Autodesk Inventor part; units mm, degrees
ref_plane "YZ Plane" through (0, 0, 0) normal (1, 0, 0) x (0, 1, 0)
ref_plane "XZ Plane" through (0, 0, 0) normal (0, 1, 0) x (-1, 0, 0)
ref_plane "XY Plane" through (0, 0, 0) normal (0, 0, 1) x (1, 0, 0)
sketch "Sketch1" plane through (0, 0, 0) normal (0, 1, 0) x (-1, 0, 0)
  circle A0 centre (0, 0) radius 53.71
  circle A1 centre (0, 0) radius 50.71
  dimension "d0" = 107.42
  dimension "d1" = 3
extrude "Extrusion1" add sketch "Sketch1" along normal blind 30
sketch "Sketch2" plane through (0, 0, 0) normal (0, -1, 0) x (1, 0, 0)
  circle A0 centre (0, 0) radius 53.71
  circle A1 centre (0, 0) radius 50.71
  circle A2 centre (0, 0) radius 40.71
  dimension "d5" = 10
extrude "Extrusion2" add sketch "Sketch2" along normal blind 3 contours A0 | A1
properties part number "12mm-CoilForm-Stiffner"
The listing builds one solid part. Answer for the finished solid, in the listing's coordinates (mm). A direction names the side the tool comes from. Round coordinates to 2 decimals unless told otherwise and drop trailing zeros. Write each loop counter-clockwise with the first axis right and the second up, starting at its lowest first coordinate (ties: lowest second). Pieces come first, ordered by that corner, then holes. Notation, with made-up numbers: (-36.5, 43.25) - (-8.5, 43.25) arc R18 ccw to (-8.5, 77.25) - close; hole circle Ø1 at (69, 0.25). An arc over 180 degrees is marked (long way). Use one line per item in the form item = value. Start each with the question number.
Item 1: A tool of negligible diameter and unlimited length cuts with its end or side. For faces 1 (the flat face through (-40, 30, 32)), 2 (the flat face through (0, 0, 42)), from which of +Z, -Z, +X, -X, +Y, -Y can it reach the whole face along a straight path? Write none if from no direction.
Item 2: Flat-ended cylindrical pins translate along their axes: pin 1 Ø10 at (y, z) = (19, 27.5) entering from +X; pin 2 Ø4 at (x, y) = (42, 11.5) entering from +Z; pin 3 Ø10 at (x, y) = (-42.5, 23) entering from -Z. Find the tip coordinate at first contact, or state that the pin passes through.
Item 3: A cutting plane is placed at D-D (x = -47). Write down the section's boundary in (y, z), plus the area to 3 significant figures.
Item 4: A cutting plane is placed at B-B (x = 0). Write down the section's boundary in (y, z).
Item 5: Determine the mould class of faces 3 (the flat face through (-8.21, -3, 40.04)), 4 (the cylindrical face through (38.83, -1.48, -12.23)) for opening direction Z: +Z half, -Z half, draft (parallel to the pull), parting line (faces both ways), or undercut.
Item 6: Find the intervals of material crossed by line 1 (Z direction, x = 0, y = -1.15); line 2 (Z direction, x = 0, y = 10); line 3 (Y direction, x = -4.5, z = -40.5), in increasing order. Write a range as [from, to].
Item 7: A cutting plane is placed at C-C (y = 25.5). Write down the section's boundary in (x, z), plus the area to 3 significant figures.
Item 8: A cutting plane is placed at A-A (z = 0). Write down the section's boundary in (x, y), plus the area to 3 significant figures.
The answers:
q1.face_1 = +Z, -Z, +X, -X, +Y
q1.face_2 = +Y
q2.pin_1 = 48.77
q2.pin_2 = 35.84
q2.pin_3 = -38.45
q3.outline = (-3, -26) - (30, -26) - (30, -19.04) - (0, -19.04) - (0, 19.04) - (30, 19.04) - (30, 26) - (-3, 26) - close
q3.area = 573 mm^2
q4.outline = (-3, -53.71) - (30, -53.71) - (30, -50.71) - (0, -50.71) - (0, -40.71) - (-3, -40.71) - close; (-3, 40.71) - (0, 40.71) - (0, 50.71) - (30, 50.71) - (30, 53.71) - (-3, 53.71) - close
q5.face_3 = draft
q5.face_4 = undercut
q6.line_1 = [-53.71, -40.71], [40.71, 53.71]
q6.line_2 = [-53.71, -50.71], [50.71, 53.71]
q6.line_3 = [-3, 0]
q7.outline = circle Ø107.42 at (0, 0); hole circle Ø101.42 at (0, 0)
q7.area = 984 mm^2
q8.outline = (-53.71, -3) - (-40.71, -3) - (-40.71, 0) - (-50.71, 0) - (-50.71, 30) - (-53.71, 30) - close; (40.71, -3) - (53.71, -3) - (53.71, 30) - (50.71, 30) - (50.71, 0) - (40.71, 0) - close
q8.area = 258 mm^2
